Read the model definition and answer for the solid it produces. Units are mm, in the model's axes. Face numbers are marked on the shaded views. A direction names the side the tool comes from. Round coordinates to 2 decimals unless told otherwise and drop trailing zeros. Loops run counter-clockwise (first coordinate to the right, second up) from the corner with the lowest first, then second, coordinate; pieces in that order, holes last. Notation, with made-up numbers: (2.5, -38) - (36.5, -38) arc R16 cw to (36.5, -21) - close; hole circle Ø10 at (-35, 9.5). An arc over 180 degrees is marked (long way). Answer as CSV lines item,"result".
```python
from build123d import *

# Parameters (mm, degrees)
BOSS_EXTRUDE1_DEPTH = 8
CHAMFER5_SIZE       = 3
FILLET1_R           = 2.5
SKETCH2_R           = 2
CUT_EXTRUDE1_DEPTH  = 63.819184968
SKETCH3_R           = 1.8
CUT_EXTRUDE2_DEPTH  = 60.634302209
SKETCH5_W           = 8.5
SKETCH5_H           = 8
CUT_EXTRUDE3_DEPTH  = 15
CUT_EXTRUDE5_DEPTH  = 15
CHAMFER6_SIZE       = 2


with BuildPart() as part:
    # Sketch1 → Boss-Extrude1 (new, symmetric)
    with BuildSketch(Plane.XY):
        Polygon((-50, 0), (-33, 0), (-33, 30), (33, 30), (33, 0), (50, 0), (50, 3), (41.5, 3), (41.5, 34.5), (-41.5, 34.5), (-41.5, 3), (-50, 3), align=None)
    extrude(amount=BOSS_EXTRUDE1_DEPTH, both=True)

    # Chamfer5
    chamfer5_edges = [part.edges().sort_by_distance(p)[0] for p in [
        (-41.5, 34.5, 0),
        (41.5, 34.5, 0),
        (33, 0, 0),
        (-33, 0, 0),
    ]]
    chamfer(chamfer5_edges, length=CHAMFER5_SIZE)

    # Fillet1
    fillet1_edges = [part.edges().sort_by_distance(p)[0] for p in [
        (-41.5, 3, 0),
        (41.5, 3, 0),
    ]]
    fillet(fillet1_edges, radius=FILLET1_R)

    # Sketch2 → Cut-Extrude1 (cut, through all)
    with BuildSketch(Plane.XY.offset(8)):
        with Locations((37, 23.5)):
            Circle(SKETCH2_R)
        with Locations((37, 6.5)):
            Circle(SKETCH2_R)
    cut_extrude1 = extrude(amount=-CUT_EXTRUDE1_DEPTH, mode=Mode.SUBTRACT)

    # Mirror1: Cut-Extrude1 across plane
    add(cut_extrude1.mirror(Plane(origin=(0, 0, 0), x_dir=(0, 0, 1), z_dir=(1, 0, 0))), mode=Mode.SUBTRACT)

    # Sketch3 → Cut-Extrude2 (cut, through all)
    with BuildSketch(Plane(origin=(0, 3, 0), x_dir=(1, 0, 0), z_dir=(0, 1, 0))):
        with Locations(Location((46, 4, 0), (0, 0, 270))):
            Circle(SKETCH3_R)
        with Locations(Location((46, -4, 0), (0, 0, 270))):
            Circle(SKETCH3_R)
        with Locations(Location((-46, 4, 0), (0, 0, 270))):
            Circle(SKETCH3_R)
        with Locations(Location((-46, -4, 0), (0, 0, 270))):
            Circle(SKETCH3_R)
    extrude(amount=-CUT_EXTRUDE2_DEPTH, mode=Mode.SUBTRACT)

    # Sketch5 → Cut-Extrude3 (cut)
    with BuildSketch(Plane(origin=(0, 34.5, 0), x_dir=(1, 0, 0), z_dir=(0, 1, 0))):
        with Locations((37.25, 0)):
            Rectangle(SKETCH5_W, SKETCH5_H)
        with Locations((-37.25, 0)):
            Rectangle(SKETCH5_W, SKETCH5_H)
    extrude(amount=-CUT_EXTRUDE3_DEPTH, mode=Mode.SUBTRACT)

    # Sketch7 → Cut-Extrude5 (cut)
    with BuildSketch(Plane(origin=(0, 34.5, 0), x_dir=(1, 0, 0), z_dir=(0, 1, 0))):
        with BuildLine():
            Line((33, 4), (33, -4))
            ThreePointArc((33, -4), (29, 0), (33, 4))
        make_face()
        with BuildLine():
            Line((-33, 4), (-33, -4))
            ThreePointArc((-33, -4), (-29, 0), (-33, 4))
        make_face()
    extrude(amount=-CUT_EXTRUDE5_DEPTH, mode=Mode.SUBTRACT)

    # Chamfer6
    chamfer6_edges = [part.edges().sort_by_distance(p)[0] for p in [
        (0, 34.5, -8),
        (0, 34.5, 8),
    ]]
    chamfer(chamfer6_edges, length=CHAMFER6_SIZE)


solid = part.part
```
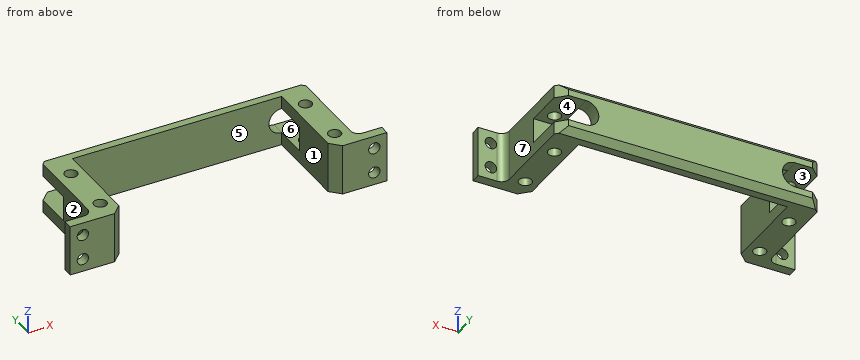
1) Find the intervals of material crossed by line 1 (Y direction, x = 37, z = -5.15); line 2 (X direction, y = 14, z = -0.25); line 3 (X direction, y = 24.5, z = 5.5), in increasing order.
Entries:
line 1,"y = 0 to 4.5, 8.5 to 21.5, 25.5 to 34.5"
line 2,"x = -41.5 to -33, 33 to 41.5"
line 3,"x = -41.5 to -38.73, -35.27 to -33, 33 to 35.27, 38.73 to 41.5"
2) A cutting plane is placed at B-B, the plane y = 26.5. Determine the outline of the cut face in (x, z).
Entries:
outline,"(-41.5, -8) - (-33, -8) - (-33, -4) - (-41.5, -4) - close; (-41.5, 4) - (-33, 4) - (-33, 8) - (-41.5, 8) - close; (33, -8) - (41.5, -8) - (41.5, -4) - (33, -4) - close; (33, 4) - (41.5, 4) - (41.5, 8) - (33, 8) - close"
3) A cutting plane is placed at A-A, the plane x = 46. Determine the outline of the cut face in (y, z), plus the area to 3 significant figures.
Entries:
outline,"(0, -8) - (3, -8) - (3, -5.8) - (0, -5.8) - close; (0, -2.2) - (3, -2.2) - (3, 2.2) - (0, 2.2) - close; (0, 5.8) - (3, 5.8) - (3, 8) - (0, 8) - close"
area,"26.4 mm^2"
4) The mould has two halves that part along X. Classify the marked faces 5, 6 and 7: pulls with the +X half, pulls with the -X half, needs draft (parallel to the pull), parting line crosses it, or undercut.
Entries:
face 5,"undercut"
face 6,"needs draft"
face 7,"pulls with the +X half"
5) A cutting plane is placed at D-D, the plane y = 17.5. Determine the outline of the cut face in (x, z).
Entries:
outline,"(-41.5, -8) - (-33, -8) - (-33, 8) - (-41.5, 8) - close; (33, -8) - (41.5, -8) - (41.5, 8) - (33, 8) - close"
6) A cutting plane is placed at C-C, the plane z = -0.25. Determine the outline of the cut face in (x, y).
Entries:
outline,"(-50, 0) - (-36, 0) - (-33, 3) - (-33, 19.5) - (-41.5, 19.5) - (-41.5, 5.5) arc R2.5 cw to (-44, 3) - (-50, 3) - close; (-29.01, 30) - (29.01, 30) - (29.01, 34.5) - (-29.01, 34.5) - close; (33, 3) - (36, 0) - (50, 0) - (50, 3) - (44, 3) arc R2.5 cw to (41.5, 5.5) - (41.5, 19.5) - (33, 19.5) - close; hole circle Ø4 at (-37, 6.5); hole circle Ø4 at (37, 6.5)"
7) A tool of negligible diameter and unlimited length cuts with its end or side. For the marked faces 1, 2, 3 and 4, from which of +Z, -Z, +X, -X, +Y, -Y can it reach the whole face along a straight path? Write none if from no direction.
Entries:
face 1,"+Z, -Z, -Y"
face 2,"+Z, -Z, -X, +Y"
face 3,"-X, +Y"
face 4,"+X, +Y"
8) Each of these flat-tipped pins is pushed along its axis until it touches: P1, Ø3, axis at x = 37, y = 6.5, coming from the +Z side; P2, Ø8, axis at y = 18.5, z = 4, coming from the +X side; P3, Ø4, axis at x = -19.5, z = 0, coming from the -Y side; P4, Ø5, axis at y = 21, z = 3, coming from the -X side. Where does it stop, or does it pass through?
Entries:
P1,"passes through"
P2,"stops at x = 41.5"
P3,"stops at y = 30"
P4,"stops at x = -41.5"
